Job drawing, mm, ordinate dimensions from the low corner. One solid piece. A direction names the side the tool comes from. Round coordinates to 2 decimals unless told otherwise and drop trailing zeros. Loops run counter-clockwise (first coordinate to the right, second up) from the corner with the lowest first, then second, coordinate; pieces in that order, holes last.
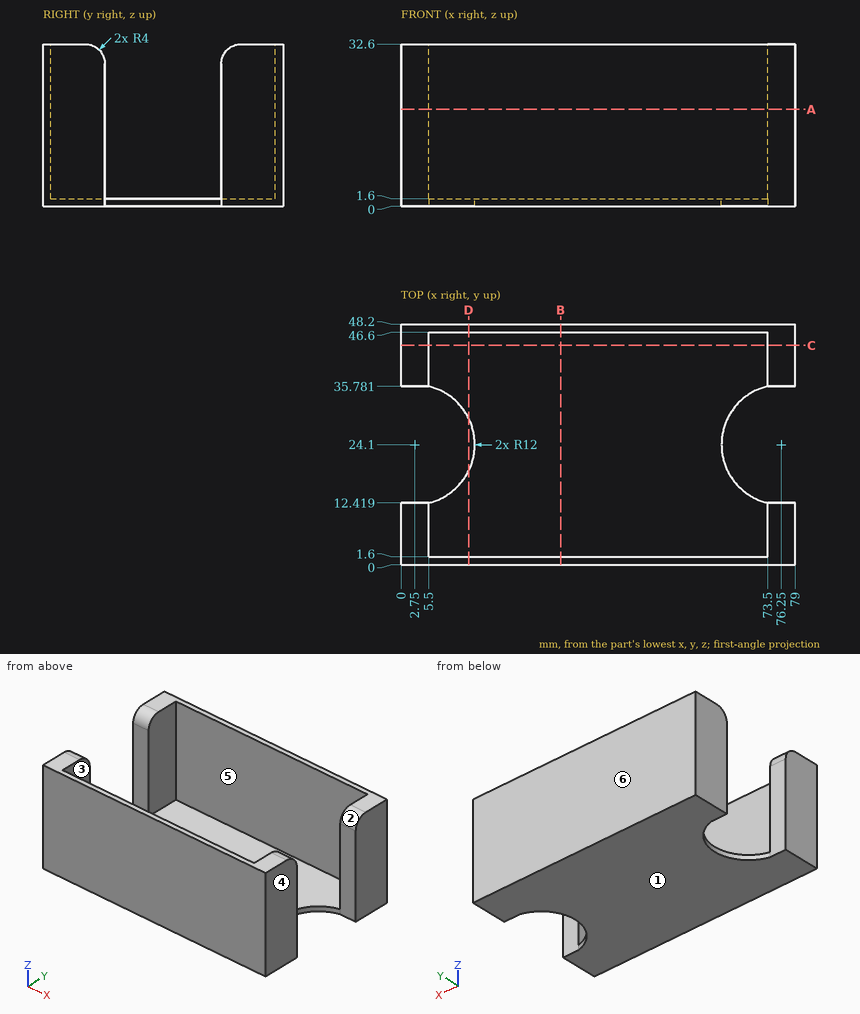
(1) Pin check, flat tips, straight feed: P1, Ø15.5, axis at x = 35.5, z = 9.5, coming from the -Y side; P2, Ø10, axis at x = 49, y = 39, coming from the +Z side. Stop position of each tip, or through.
Responses:
P1: stops at y = 0
P2: stops at z = 1.6
(2) Slice it at A-A on z = 19.5. List the corners of the cut face in (x, y), plus the area to 3 significant figures.
Responses:
outline: (0, 0) - (79, 0) - (79, 12.42) - (73.5, 12.42) - (73.5, 1.6) - (5.5, 1.6) - (5.5, 12.42) - (0, 12.42) - close; (0, 35.78) - (5.5, 35.78) - (5.5, 46.6) - (73.5, 46.6) - (73.5, 35.78) - (79, 35.78) - (79, 48.2) - (0, 48.2) - close
area: 491 mm2
(3) Which spindle directions (+Z, -Z, +X, -X, +Y, -Y) get a long thin tool onto all of the face, cutting with end or side? Do the marked faces 1, 2 and 3. Say none if no direction does.
Responses:
face 1: -Z, +X, -X, +Y, -Y
face 2: +Z, +X, -X
face 3: +Z
(4) Slice it at B-B on x = 32. List the corners of the cut face in (y, z), plus the area to 3 significant figures.
Responses:
outline: (0, 0) - (48.2, 0) - (48.2, 32.6) - (46.6, 32.6) - (46.6, 1.6) - (1.6, 1.6) - (1.6, 32.6) - (0, 32.6) - close
area: 176 mm2
(5) Slice it at D-D on x = 13.5. List the corners of the cut face in (y, z), plus the area to 3 significant figures.
Responses:
outline: (0, 0) - (18.77, 0) - (18.77, 1.6) - (1.6, 1.6) - (1.6, 32.6) - (0, 32.6) - close; (29.43, 0) - (48.2, 0) - (48.2, 32.6) - (46.6, 32.6) - (46.6, 1.6) - (29.43, 1.6) - close
area: 159 mm2
(6) Slice it at C-C on y = 44. List the corners of the cut face in (x, z).
Responses:
outline: (0, 0) - (79, 0) - (79, 32.6) - (73.5, 32.6) - (73.5, 1.6) - (5.5, 1.6) - (5.5, 32.6) - (0, 32.6) - close
(7) Probe line 1 (Y direction, x = 3.5, z = 2.5); line 2 (Y direction, x = 38.5, z = 31); line 3 (X direction, y = 41, z = 23.5). List the from-to ranges inside material, lowest first.
Responses:
line 1: y = 0 to 12.42, 35.78 to 48.2
line 2: y = 0 to 1.6, 46.6 to 48.2
line 3: x = 0 to 5.5, 73.5 to 79
(8) Pull direction Y, two halves, no side cores. Call the marked faces 4, 5 and 6: +Y half, -Y half, draft (parallel to the pull), parting line (faces both ways), or undercut.
Responses:
face 4: draft
face 5: undercut
face 6: +Y half
